For this review, take the finished solid that the model builds, in its own axes (mm). A direction names the side the tool comes from. Coordinates: 2 decimals unless noted, no trailing zeros. Write each loop counter-clockwise with the first axis right and the second up, starting at its lowest first coordinate (ties: lowest second). Pieces come first, ordered by that corner, then holes. Notation, with made-up numbers: (-22, -20.75) -> (-13, -20.75) arc R16 cw to (-13, 5.25) -> close; hole circle Ø9 at (-6, 11). An arc over 180 degrees is marked (long way). Put each result on its own line as item: value. Start each with the question number.
Item 1: Consider section C-C on z = 15.5. Give the boundary of the cut face in (x, y).
Item 2: To check wall thickness, follow L1, parallel to X at y = -72, z = 0.5. State the ranges of the line that lie inside material, in increasing order.
Item 3: The part is to be moulded in two halves that separate along Z. For faces 1 (the flat face through (0, -46, 18)), 2 (the flat face through (0, -46, 20)), 3 (the flat face through (18, -46, 0)), 4 (the flat face through (-20, -46, 0)), say which applies: +Z half, -Z half, draft (parallel to the pull), parting line (faces both ways), or undercut.
Item 4: For faces 5 (the cylindrical face through (0, -5, 19)), 6 (the flat face through (-18, -46, 0)), list the 3-axis set-ups (+Z, -Z, +X, -X, +Y, -Y) from which the entire face can be reached by the end or side of a thin tool; tool diameter is ignored.
Item 5: Consider section B-B on y = -78.5. Give the boundary of the cut face in (x, z).
Item 6: Consider section A-A on x = -15.5. Give the boundary of the cut face in (y, z).
```python
from build123d import *

# Parameters (mm, degrees)
ESBO_O1_W             = 40
ESBO_O1_H             = 40
ESBO_O1_W_2           = 36
ESBO_O1_H_2           = 36
ESBO_O3_R             = 15
CORTE_EXTRUS_O1_DEPTH = 50


with BuildPart() as part:
    # Varredura1: sweep along a path in Esboço2
    with BuildLine(Plane(origin=(0, 0, 0), x_dir=(0, 0, -1), z_dir=(1, 0, 0))) as varredura1_path:
        Line((0, 0), (0, -90))
    # Esboço1 → Varredura1 (sweep)
    with BuildSketch(Plane(origin=(0, 0, 0), x_dir=(1, 0, 0), z_dir=(0, 1, 0))):
        Rectangle(ESBO_O1_W, ESBO_O1_H)
        Rectangle(ESBO_O1_W_2, ESBO_O1_H_2, mode=Mode.SUBTRACT)
    sweep(path=varredura1_path.line)

    # Esboço3 → Corte-extrusão1 (cut)
    with BuildSketch(Plane.XY.offset(20)):
        with Locations((0, 10)):
            Circle(ESBO_O3_R)
    extrude(amount=-CORTE_EXTRUS_O1_DEPTH, mode=Mode.SUBTRACT)


solid = part.part
```
Return value:
1. outline: (-20, -90) -> (-18, -90) -> (-18, 0) -> (-20, 0) -> close; (18, -90) -> (20, -90) -> (20, 0) -> (18, 0) -> close
2. L1: -20 to -18, 18 to 20
3. face 1: undercut
3. face 2: +Z half
3. face 3: undercut
3. face 4: draft
4. face 5: +Z, -Z, +Y
4. face 6: +Y, -Y
5. outline: (-20, -20) -> (20, -20) -> (20, 20) -> (-20, 20) -> close; hole (-18, -18) -> (18, -18) -> (18, 18) -> (-18, 18) -> close
6. outline: (-90, -20) -> (0, -20) -> (0, -18) -> (-90, -18) -> close; (-90, 18) -> (0, 18) -> (0, 20) -> (-90, 20) -> close
